Here's how the part is built. I have some questions about the finished solid (model axes, mm). Face numbers are marked on the shaded views. Give positions to 0.01 mm unless a question says otherwise; leave off trailing zeros. Write each loop counter-clockwise with the first axis right and the second up, starting at its lowest first coordinate (ties: lowest second). Pieces come first, ordered by that corner, then holes. Notation, with made-up numbers: (69, 33.5) -> (82, 33.5) arc R17 ccw to (82, 56.5) -> close; hole circle Ø7 at (74, -24.75). An arc over 180 degrees is marked (long way). Use one line per item in the form item = value.
```python
from build123d import *

# Parameters (mm, degrees)
SKETCH_1_W          = 210
SKETCH_1_H          = 76.65
SKETCH_1_W_2        = 170
SKETCH_1_H_2        = 46.1
EXTRUDE_1_DEPTH     = 13
SKETCH_2_W          = 210
SKETCH_2_H          = 68
CUT_EXTRUDE_1_DEPTH = 9
CHAMFER_1_SIZE      = 1
EXTRUDE_2_DEPTH     = 210
SKETCH_7_W          = 20
SKETCH_7_H          = 76.65
CUT_EXTRUDE_2_DEPTH = 4.9


with BuildPart() as part:
    # 草图1 → 凸台-拉伸1 (new body)
    with BuildSketch(Plane.XY):
        Rectangle(SKETCH_1_W, SKETCH_1_H)
        with Locations((0, -2.325)):
            Rectangle(SKETCH_1_W_2, SKETCH_1_H_2, mode=Mode.SUBTRACT)
    extrude(amount=EXTRUDE_1_DEPTH)

    # 草图2 → 切除-拉伸1 (cut)
    with BuildSketch(Plane.XY.offset(13)):
        Rectangle(SKETCH_2_W, SKETCH_2_H)
    extrude(amount=-CUT_EXTRUDE_1_DEPTH, mode=Mode.SUBTRACT)

    # 倒角1
    chamfer_1_edges = [part.edges().sort_by_distance(p)[0] for p in [
        (105, -36.1625, 13),
        (0, 38.325, 13),
        (105, 36.1625, 13),
        (-105, -36.1625, 13),
        (-105, 36.1625, 13),
        (0, -38.325, 13),
    ]]
    chamfer(chamfer_1_edges, length=CHAMFER_1_SIZE)

    # 草图6 → 凸台-拉伸2 (add)
    with BuildSketch(Plane(origin=(105, 0, 0), x_dir=(0, 0, -1), z_dir=(1, 0, 0))):
        Polygon((0, 20.725), (0, 26.625), (1.9, 26.625), (1.9, 28.975), (3.4, 28.975), (4.9, 27.475), (4.9, 19.875), (3.4, 18.375), (1.9, 18.375), (1.9, 20.725), align=None)
        Polygon((0, -31.275), (0, -25.375), (1.9, -25.375), (1.9, -23.025), (3.4, -23.025), (4.9, -24.525), (4.9, -32.125), (3.4, -33.625), (1.9, -33.625), (1.9, -31.275), align=None)
    extrude(amount=-EXTRUDE_2_DEPTH)

    # 草图7 → 切除-拉伸2 (cut)
    with BuildSketch(Plane(origin=(0, 0, -4.9), x_dir=(-1, 0, 0), z_dir=(0, 0, -1))):
        with Locations((-95, 0)):
            Rectangle(SKETCH_7_W, SKETCH_7_H)
        with Locations((95, 0)):
            Rectangle(SKETCH_7_W, SKETCH_7_H)
    extrude(amount=-CUT_EXTRUDE_2_DEPTH, mode=Mode.SUBTRACT)


solid = part.part
```
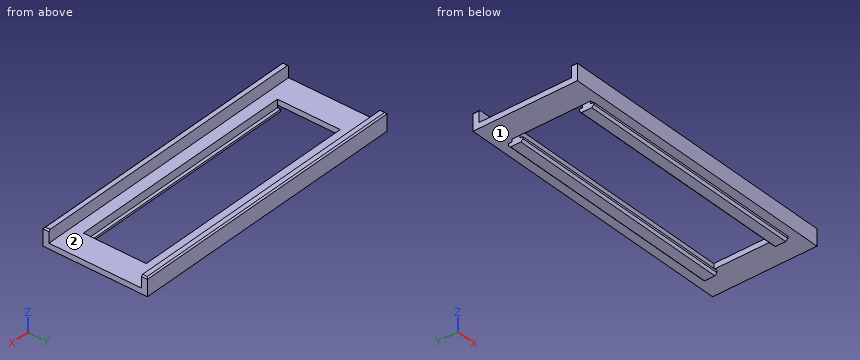
Q1. If we mould it in two halves opening along Y, with no side actions, what happens to the marked faces 1 and 2? For each: +Y half, -Y half, draft (parallel to the pull), parting line (faces both ways), or undercut.
Result set:
face_1 = draft
face_2 = undercut
Q2. I want a section at B-B, the plane y = 11.5. Write out the boundary of the cut face in (x, z).
Result set:
outline = (-105, 0) -> (-85, 0) -> (-85, 4) -> (-105, 4) -> close; (85, 0) -> (105, 0) -> (105, 4) -> (85, 4) -> close
Q3. If I drill on line 1 along Y through (x, z) = (45.5, 6.5) (3 decimals); line 2 along X through (y, z) = (2, 3.25); line 3 along Z through (x, y) = (-27, 27), over which ranges is the centre line in solid material (lowest first)? Write a range as from..to.
Result set:
line_1 = -38.325..-34, 34..38.325
line_2 = -105..-85, 85..105
line_3 = -4.9..-1.9, 0..4
Q4. I want a section at C-C, the plane z = 8. Write out the boundary of the cut face in (x, y) (3 decimals), and give its area (3 significant figures).
Result set:
outline = (-105, -38.325) -> (105, -38.325) -> (105, -34) -> (-105, -34) -> close; (-105, 34) -> (105, 34) -> (105, 38.325) -> (-105, 38.325) -> close
area = 1,820 mm2
Q5. Will these pins go through, and if not, where does the flat tip stop? pin 1 Ø5.5 at (y, z) = (24, -2) entering from -X; pin 2 Ø0.7 at (x, y) = (40.5, -32.5) entering from +Z; pin 3 Ø20.5 at (x, y) = (35.5, -1) entering from +Z; pin 4 Ø0.8 at (x, z) = (15, -2.5) entering from -Y (3 decimals).
Result set:
pin_1 = -105
pin_2 = 4
pin_3 = through
pin_4 = -33.625
